The listing builds one solid part. Answer for the finished solid, in the listing's coordinates (mm). A direction names the side the tool comes from. Give positions to 0.01 mm unless a question says otherwise; leave off trailing zeros. Write each loop counter-clockwise with the first axis right and the second up, starting at its lowest first coordinate (ties: lowest second). Pieces come first, ordered by that corner, then holes. Notation, with made-up numbers: (60, -3) -> (98, -3) arc R35 ccw to (98, 34) -> close; hole circle Ø11 at (4, 63.5). An arc over 180 degrees is marked (long way). Write each question's results on one line, items separated by ' | '. Start each with the question number.
from build123d import *

# Parameters (mm, degrees)
SKETCH1_W           = 94
SKETCH1_H           = 74
BOSS_EXTRUDE1_DEPTH = 12
SKETCH2_W           = 90.5
SKETCH2_H           = 70.5
CUT_EXTRUDE1_DEPTH  = 3.5
SKETCH3_R           = 1.5
CUT_EXTRUDE2_DEPTH  = 6
SHELL1_START        = 3
SHELL1_DEPTH        = 5.5
CHAMFER1_SIZE       = 1
CHAMFER2_SIZE       = 1
CHAMFER3_SIZE       = 1
SKETCH4_R           = 2.1
CUT_EXTRUDE3_DEPTH  = 61.489668539


# Read off the part's stored shape, not the designer's step: Shell1
with BuildPart() as part:
    # Sketch1 → Boss-Extrude1 (new body)
    with BuildSketch(Plane(origin=(0, 0, 0), x_dir=(1, 0, 0), z_dir=(0, 1, 0))):
        Rectangle(SKETCH1_W, SKETCH1_H)
    extrude(amount=BOSS_EXTRUDE1_DEPTH)

    # Sketch2 → Cut-Extrude1 (cut)
    with BuildSketch(Plane(origin=(0, 12, 0), x_dir=(1, 0, 0), z_dir=(0, 1, 0))):
        Rectangle(SKETCH2_W, SKETCH2_H)
    extrude(amount=-CUT_EXTRUDE1_DEPTH, mode=Mode.SUBTRACT)

    # Sketch3 → Cut-Extrude2 (cut)
    with BuildSketch(Plane(origin=(0, 8.5, 0), x_dir=(1, 0, 0), z_dir=(0, 1, 0))):
        with Locations(Location((-42.5, 33.055555556, 0), (0, 0, 270))):
            Circle(SKETCH3_R)
        with Locations(Location((42.5, 33.055555556, 0), (0, 0, 270))):
            Circle(SKETCH3_R)
        with Locations(Location((42.5, -33.055555556, 0), (0, 0, 270))):
            Circle(SKETCH3_R)
        with Locations(Location((-42.5, -33.055555556, 0), (0, 0, 270))):
            Circle(SKETCH3_R)
    extrude(amount=-CUT_EXTRUDE2_DEPTH, mode=Mode.SUBTRACT)

    # Shell1 outline → Shell1 (cut)
    with BuildSketch(Plane(origin=(0, 0, 0), x_dir=(1, 0, 0), z_dir=(0, 1, 0)).offset(SHELL1_START)):
        with BuildLine():
            Line((-38.100224473, -34), (38.100224473, -34))
            ThreePointArc((38.100224473, -34), (39.528697665, -29.67600493), (44, -28.812914868))
            Line((44, -28.812914868), (44, 28.812914868))
            ThreePointArc((44, 28.812914868), (39.528697665, 29.67600493), (38.100224473, 34))
            Line((38.100224473, 34), (-38.100224473, 34))
            ThreePointArc((-38.100224473, 34), (-39.528697665, 29.67600493), (-44, 28.812914868))
            Line((-44, 28.812914868), (-44, -28.812914868))
            ThreePointArc((-44, -28.812914868), (-39.528697665, -29.67600493), (-38.100224473, -34))
        make_face()
    extrude(amount=SHELL1_DEPTH, mode=Mode.SUBTRACT)

    # Chamfer1
    chamfer1_edges = [part.edges().sort_by_distance(p)[0] for p in [
        (45.25, 12, 0),
        (0, 12, -35.25),
        (-45.25, 12, 0),
        (0, 12, 35.25),
    ]]
    chamfer(chamfer1_edges, length=CHAMFER1_SIZE)

    # Chamfer2
    chamfer2_edges = [part.edges().sort_by_distance(p)[0] for p in [
        (0, 8.5, 34),
        (44, 8.5, 0),
        (0, 8.5, -34),
        (-44, 8.5, 0),
        (-39.528697665, 8.5, -29.67600493),
        (39.528697665, 8.5, -29.67600493),
        (39.528697665, 8.5, 29.67600493),
        (-39.528697665, 8.5, 29.67600493),
    ]]
    chamfer(chamfer2_edges, length=CHAMFER2_SIZE)

    # Chamfer3
    chamfer3_edges = [part.edges().sort_by_distance(p)[0] for p in [
        (-47, 6, 37),
        (-47, 6, -37),
        (47, 6, -37),
        (47, 6, 37),
    ]]
    chamfer(chamfer3_edges, length=CHAMFER3_SIZE)

    # Sketch4 → Cut-Extrude3 (cut, through all)
    with BuildSketch(Plane(origin=(0, 3, 0), x_dir=(1, 0, 0), z_dir=(0, 1, 0))):
        with Locations(Location((-10.4, 0, 0), (0, 0, 270))):
            Circle(SKETCH4_R)
        with Locations(Location((10.4, 0, 0), (0, 0, 270))):
            Circle(SKETCH4_R)
    extrude(amount=-CUT_EXTRUDE3_DEPTH, mode=Mode.SUBTRACT)


solid = part.part
1. Section D-D (x = 42.5) is taken. Write down the section's boundary in (y, z), then the cut area to 3 significant figures.
2. Section B-B (z = 0) is taken. Write down the section's boundary in (x, y).
3. Each of these flat-tipped pins is pushed along its axis until it touches: pin 1 Ø1.5 at (x, z) = (-42, 33.5) entering from +Y; pin 2 Ø4 at (x, z) = (10.4, 0) entering from -Y; pin 3 Ø2.5 at (x, z) = (43, -32.5) entering from +Y; pin 4 Ø21 at (x, z) = (-16.5, -11) entering from +Y. Where does it stop, or does it pass through?
4. Section C-C (y = 5) is taken. Write down the section's boundary in (x, z), then the cut area to 3 significant figures.
5. A tool of negligible diameter and unlimited length cuts with its end or side. For faces 1 (the flat face through (-1, 10, -35.25)), 2 (the cylindrical face through (-8.318, 1.521, -0.273)), from which of +Z, -Z, +X, -X, +Y, -Y can it reach the whole face along a straight path? Write none if from no direction.
6. Section A-A (x = -10.4) is taken. Write down the section's boundary in (y, z), then the cut area to 3 significant figures.
7. The mould has two halves that part along X. Classify faces 3 (the flat face through (-1, 6, -37)), 4 (the conical face through (-40.13, 8.33, -30.25)): pulls with the +X half, pulls with the -X half, needs draft (parallel to the pull), parting line crosses it, or undercut.
8. Consider probe 1 along X at (y, z) = (0.7, 0); probe 2 along Z at (x, y) = (20, 4.25); probe 3 along X at (y, z) = (4, -8). Determine where each line is inside the solid, lowest interval first. Write a range as [from, to].
Results:
1) outline: (0, -37) -> (12, -37) -> (12, -36.25) -> (11, -35.25) -> (8.5, -35.25) -> (8.5, -34.56) -> (2.5, -34.56) -> (2.5, -31.56) -> (8.5, -31.56) -> (8.5, -29.56) -> (7.5, -28.56) -> (3, -28.56) -> (3, 28.56) -> (7.5, 28.56) -> (8.5, 29.56) -> (8.5, 31.56) -> (2.5, 31.56) -> (2.5, 34.56) -> (8.5, 34.56) -> (8.5, 35.25) -> (11, 35.25) -> (12, 36.25) -> (12, 37) -> (0, 37) -> close | area: 289 mm²
2) outline: (-47, 0) -> (-12.5, 0) -> (-12.5, 3) -> (-44, 3) -> (-44, 7.5) -> (-45, 8.5) -> (-45.25, 8.5) -> (-45.25, 11) -> (-46.25, 12) -> (-47, 12) -> close; (-8.3, 0) -> (8.3, 0) -> (8.3, 3) -> (-8.3, 3) -> close; (12.5, 0) -> (47, 0) -> (47, 12) -> (46.25, 12) -> (45.25, 11) -> (45.25, 8.5) -> (45, 8.5) -> (44, 7.5) -> (44, 3) -> (12.5, 3) -> close
3) pin 1: stops at y = 2.5 | pin 2: passes through | pin 3: stops at y = 8.5 | pin 4: stops at y = 3
4) outline: (-47, -36) -> (-46, -37) -> (46, -37) -> (47, -36) -> (47, 36) -> (46, 37) -> (-46, 37) -> (-47, 36) -> close; hole circle Ø3 at (-42.5, -33.06); hole (-44, -28.81) arc R4.5 cw to (-38.1, -34) -> (38.1, -34) arc R4.5 cw to (44, -28.81) -> (44, 28.81) arc R4.5 cw to (38.1, 34) -> (-38.1, 34) arc R4.5 cw to (-44, 28.81) -> close; hole circle Ø3 at (-42.5, 33.06); hole circle Ø3 at (42.5, -33.06); hole circle Ø3 at (42.5, 33.06) | area: 1,050 mm²
5) face 1: +Y | face 2: +Y, -Y
6) outline: (0, -37) -> (12, -37) -> (12, -36.25) -> (11, -35.25) -> (8.5, -35.25) -> (8.5, -35) -> (7.5, -34) -> (3, -34) -> (3, -2.1) -> (0, -2.1) -> close; (0, 2.1) -> (3, 2.1) -> (3, 34) -> (7.5, 34) -> (8.5, 35) -> (8.5, 35.25) -> (11, 35.25) -> (12, 36.25) -> (12, 37) -> (0, 37) -> close | area: 253 mm²
7) face 3: needs draft | face 4: undercut
8) probe 1: x = [-47, -12.5], [-8.3, 8.3], [12.5, 47] | probe 2: z = [-37, -34], [34, 37] | probe 3: x = [-47, -44], [44, 47]
